Read the model definition and answer for the solid it produces. Units are mm, in the model's axes. Give positions to 0.01 mm unless a question says otherwise; leave off trailing zeros. Order: outer loops, then holes, each group sorted by start corner. A loop starts at its lowest first (then second) coordinate and runs counter-clockwise, first axis right, second up.
```python
from build123d import *

# Parameters (mm, degrees)
SKETCH1_W                = 50
SKETCH1_H                = 27
BOSS_EXTRUDE1_DEPTH      = 3
FILLET1_R                = 25
M4_CLEARANCE_HOLE2_D     = 4.5
M4_CLEARANCE_HOLE2_DEPTH = 3
M4_CLEARANCE_HOLE2_TIP   = 1.351936393


with BuildPart() as part:
    # Sketch1 → Boss-Extrude1 (new body)
    with BuildSketch(Plane(origin=(0, 0, 0), x_dir=(1, 0, 0), z_dir=(0, 1, 0))):
        with Locations((25, 13.5)):
            Rectangle(SKETCH1_W, SKETCH1_H)
    extrude(amount=BOSS_EXTRUDE1_DEPTH)

    # Fillet1
    fillet1_edges = [part.edges().sort_by_distance(p)[0] for p in [
        (50, 1.5, 0),
        (0, 1.5, 0),
    ]]
    fillet(fillet1_edges, radius=FILLET1_R - 0.0001)  # a hair under: the kernel refuses the full size

    # M4 Clearance Hole2
    with Locations(Plane(origin=(0, 3, 0), x_dir=(1, 0, 0), z_dir=(0, 1, 0))):
        with Locations((25, 20)):
            Hole(M4_CLEARANCE_HOLE2_D / 2, depth=M4_CLEARANCE_HOLE2_DEPTH)
            with Locations((0, 0, -(M4_CLEARANCE_HOLE2_DEPTH + M4_CLEARANCE_HOLE2_TIP / 2))):  # 118° drill point
                Cone(0, M4_CLEARANCE_HOLE2_D / 2, M4_CLEARANCE_HOLE2_TIP, mode=Mode.SUBTRACT)


solid = part.part
```
1) For a pull along Z with two mould halves and no side action, classify faces 1 (the face through (23.962, 1.479, -18.004)), 2 (the face through (50, 1, -26)), 3 (the face through (42.482, 1.521, -7.129)), 4 (the face through (25, 1, -27)) as released by +Z, released by -Z, zero draft, split by the parting line, or undercut.
Final values:
face 1: undercut
face 2: zero draft
face 3: released by +Z
face 4: released by -Z
2) Consider L1, parallel to Z at x = 25, y = 0.8; L2, parallel to X at y = 1.75, z = -20; L3, parallel to Z at x = 34, y = 2.4. Determine where each line is inside the solid, lowest interval first.
Final values:
L1: z = -27 to -22.25, -17.75 to 0
L2: x = 0.51 to 22.75, 27.25 to 49.49
L3: z = -27 to -1.68
3) The part is cut by section C-C on z = -20. Determine the outline of the cut face in (x, y), and give its area (3 significant figures).
Final values:
outline: (0.51, 0) - (22.75, 0) - (22.75, 3) - (0.51, 3) - close; (27.25, 0) - (49.49, 0) - (49.49, 3) - (27.25, 3) - close
area: 133 mm2
4) The part is cut by section B-B on x = 24. Determine the outline of the cut face in (y, z).
Final values:
outline: (0, -27) - (3, -27) - (3, -22.02) - (0, -22.02) - close; (0, -17.98) - (3, -17.98) - (3, -0.02) - (0, -0.02) - close
5) Given pin 1 (1.5 mm diameter, centred on y = 1, z = -8.5, fed in from +X); pin 2 (1 mm diameter, centred on y = 2, z = -17, fed in from +X), each flat-ended and moving along its own axis, determine where each tip first touches the part or whether it passes through.
Final values:
pin 1: stops at x = 44.41
pin 2: stops at x = 48.85
6) The part is cut by section D-D on z = -4.75. Determine the outline of the cut face in (x, y).
Final values:
outline: (10.34, 0) - (39.66, 0) - (39.66, 3) - (10.34, 3) - close
